Geometry check sheet. Reference: the model listing, model coordinates, mm. A direction names the side the tool comes from. Give positions to 0.01 mm unless a question says otherwise; leave off trailing zeros. Write each loop counter-clockwise with the first axis right and the second up, starting at its lowest first coordinate (ties: lowest second). Pieces come first, ordered by that corner, then holes. Notation, with made-up numbers: (37, 42) - (90, 42) arc R32 cw to (90, 71) - close; hole circle Ø2 at (-30, -25). An arc over 180 degrees is marked (long way). Use a Markdown table: item, result.
```python
from build123d import *
from build123d import SkipClean  # not in build123d's __all__

# Parameters (mm, degrees)
F0_W          = 30
F0_H          = 37
F0_W_2        = 3
F0_H_2        = 35
F1_DEPTH      = 32
F2_DEPTH      = 25
F3_W          = 3
F3_H          = 35
F4_DEPTH      = 30
F5_W          = 11.5
F5_H          = 11.5
F6_DEPTH      = 2
F5_R          = 2.5
F7_DEPTH      = 25
F8_T4_DEPTH   = 21.8227903205
F8_T9_DEPTH   = 21.8227903205
F8_T14_DEPTH  = 21.8227903205
F8_T19_DEPTH  = 21.8227903205
F9_R          = 7.5
F9_R_2        = 2.5
F10_DEPTH     = 3
F11_SIZE      = 2.99999
F12_W         = 11.5
F12_H         = 11.5
F13_DEPTH     = 2
F14_T4_DEPTH  = 21.8227903205
F14_T9_DEPTH  = 21.8227903205
F14_T14_DEPTH = 21.8227903205
F14_T19_DEPTH = 21.8227903205
F12_R         = 2.5
F15_DEPTH     = 25
F16_R         = 7.5
F16_R_2       = 2.5
F17_DEPTH     = 3
F19_SIZE2     = 2.99999
F19_SIZE      = 1.99999
F19_2_SIZE2   = 2.99999
F19_2_SIZE    = 1.99999
F21_DEPTH     = 5
F22_R         = 1


# Not quite as in the source:
# - a fillet or chamfer that OpenCascade refuses, or shapes differently, is made with other operations: its cross-section is extruded or revolved along the edge and cut away or added
# - a fillet or chamfer is up to 0.001 mm smaller than in the source, because OpenCascade refuses the exact size
# - after a boolean that leaves OpenCascade's solid faulty, fix() repairs it


with BuildPart() as f1:
    # F0 (on Front) → F1 (new body)
    with BuildSketch(Plane.XZ):
        with Locations((3.5, 0)):
            Rectangle(F0_W, F0_H)
        Polygon((-18.5, -18.5), (-11.5, -18.5), (-11.5, 18.5), (-13.5, 18.5), (-13.5, -16.5), (-16.5, -16.5), (-16.5, 18.5), (-18.5, 18.5), align=None)
        with Locations((-15, 1)):
            Rectangle(F0_W_2, F0_H_2)
    extrude(amount=F1_DEPTH)

    # F0 (on Front) → F2 (cut)
    with BuildSketch(Plane.XZ):
        with Locations((3.5, 0)):
            Rectangle(F0_W, F0_H)
        with Locations((-15, 1)):
            Rectangle(F0_W_2, F0_H_2)
    extrude(amount=F2_DEPTH, mode=Mode.SUBTRACT)

    # F3 (on face) → F4 (cut)
    with BuildSketch(Plane.YZ.offset(18.5)):
        with Locations((-28.5, 1)):
            Rectangle(F3_W, F3_H)
    extrude(amount=-F4_DEPTH, mode=Mode.SUBTRACT)

    # F5 (on face) → F6 (join)
    with BuildSketch(Plane(origin=(0, -25, 0), x_dir=(-1, 0, 0), z_dir=(0, 1, 0))):
        with Locations((-3.5, 1)):
            Rectangle(F5_W, F5_H)
        Polygon((-8.1188021535, 1), (-5.8094010768, 5), (-1.1905989232, 5), (1.1188021535, 1), (-1.1905989232, -3), (-5.8094010768, -3), align=None, mode=Mode.SUBTRACT)
    extrude(amount=F6_DEPTH)

    # F5 (on face) → F7 (cut)
    with BuildSketch(Plane(origin=(0, -25, 0), x_dir=(-1, 0, 0), z_dir=(0, 1, 0))):
        with Locations((-3.5, 1)):
            Circle(F5_R)
    extrude(amount=-F7_DEPTH, mode=Mode.SUBTRACT)

    # F8: chamfer of 1.5 x 2 on 4 edges, made by hand


with BuildPart() as f8_tool2:
    # F8_s3 → F8_t4 (new body)
    with BuildSketch(Plane.XY.offset(11.9113951602)):
        Polygon((9.25, -25), (7.75, -23), (9.25, -23), align=None)
    extrude(amount=-F8_T4_DEPTH)

    split(bisect_by=Plane.XZ.offset(25), keep=Keep.BOTTOM)


with BuildPart() as f1_1:
    add(f1.part, clean=False)

    # F8_t1: cut F8_tool2
    add(f8_tool2.part, mode=Mode.SUBTRACT)


with BuildPart() as f8_tool7:
    # F8_s8 → F8_t9 (new body)
    with BuildSketch(Plane.YZ.offset(-7.4113951602)):
        Polygon((-25, 6.75), (-23, 5.25), (-23, 6.75), align=None)
    extrude(amount=F8_T9_DEPTH)

    split(bisect_by=Plane.XZ.offset(25), keep=Keep.BOTTOM)


with BuildPart() as f1_2:
    add(f1_1.part, clean=False)

    # F8_t6: cut F8_tool7
    add(f8_tool7.part, mode=Mode.SUBTRACT)


with BuildPart() as f8_tool12:
    # F8_s13 → F8_t14 (new body)
    with BuildSketch(Plane.XY.offset(-9.9113951602)):
        Polygon((-2.25, -25), (-0.75, -23), (-2.25, -23), align=None)
    extrude(amount=F8_T14_DEPTH)

    split(bisect_by=Plane.XZ.offset(25), keep=Keep.BOTTOM)


with BuildPart() as f1_3:
    add(f1_2.part, clean=False)

    # F8_t11: cut F8_tool12
    add(f8_tool12.part, mode=Mode.SUBTRACT)


with BuildPart() as f8_tool17:
    # F8_s18 → F8_t19 (new body)
    with BuildSketch(Plane.YZ.offset(14.4113951602)):
        Polygon((-25, -4.75), (-23, -3.25), (-23, -4.75), align=None)
    extrude(amount=-F8_T19_DEPTH)

    split(bisect_by=Plane.XZ.offset(25), keep=Keep.BOTTOM)


with BuildPart() as f1_4:
    add(f1_3.part, clean=False)

    # F8_t16: cut F8_tool17
    add(f8_tool17.part, mode=Mode.SUBTRACT)

    # F9 (on face) → F10 (join)
    with BuildSketch(Plane.XZ.offset(32)):
        with Locations((3.5, 1)):
            Circle(F9_R)
        with Locations((3.5, 1)):
            Circle(F9_R_2, mode=Mode.SUBTRACT)
    with SkipClean():  # cleaning this boolean's faces spoils the solid; the shape is the same uncleaned
        extrude(amount=F10_DEPTH)

    # F11 (size 3 in the source; OpenCascade refuses exactly that, so slightly less here)
    f11_edges = [f1_4.edges().sort_by_distance(p)[0] for p in [
        (1, -35, 1),
    ]]
    chamfer(f11_edges, length=F11_SIZE)

    # F12 (on face) → F13 (join)
    with BuildSketch(Plane.YZ.offset(-11.5)):
        with Locations((-10, 1)):
            Rectangle(F12_W, F12_H)
        Polygon((-10, 5.6188021535), (-6, 3.3094010768), (-6, -1.3094010768), (-10, -3.6188021535), (-14, -1.3094010768), (-14, 3.3094010768), align=None, mode=Mode.SUBTRACT)
    extrude(amount=F13_DEPTH)

    add(f1_4.part.fix(), mode=Mode.REPLACE)

    # F14: chamfer of 1.5 x 2 on 4 edges, made by hand


with BuildPart() as f14_tool2:
    # F14_s3 → F14_t4 (new body)
    with BuildSketch(Plane.XY.offset(-9.9113951602)):
        Polygon((-11.5, -4.25), (-9.5, -5.75), (-9.5, -4.25), align=None)
    extrude(amount=F14_T4_DEPTH)

    split(bisect_by=Plane.YZ.offset(-11.5), keep=Keep.TOP)


with BuildPart() as f1_5:
    add(f1_4.part, clean=False)

    # F14_t1: cut F14_tool2
    add(f14_tool2.part, mode=Mode.SUBTRACT)


with BuildPart() as f14_tool7:
    # F14_s8 → F14_t9 (new body)
    with BuildSketch(Plane.XZ.offset(20.9113951602)):
        Polygon((-11.5, -4.75), (-9.5, -3.25), (-9.5, -4.75), align=None)
    extrude(amount=-F14_T9_DEPTH)

    split(bisect_by=Plane.YZ.offset(-11.5), keep=Keep.TOP)


with BuildPart() as f1_6:
    add(f1_5.part, clean=False)

    # F14_t6: cut F14_tool7
    add(f14_tool7.part, mode=Mode.SUBTRACT)


with BuildPart() as f14_tool12:
    # F14_s13 → F14_t14 (new body)
    with BuildSketch(Plane.XY.offset(11.9113951602)):
        Polygon((-11.5, -15.75), (-9.5, -14.25), (-9.5, -15.75), align=None)
    extrude(amount=-F14_T14_DEPTH)

    split(bisect_by=Plane.YZ.offset(-11.5), keep=Keep.TOP)


with BuildPart() as f1_7:
    add(f1_6.part, clean=False)

    # F14_t11: cut F14_tool12
    add(f14_tool12.part, mode=Mode.SUBTRACT)


with BuildPart() as f14_tool17:
    # F14_s18 → F14_t19 (new body)
    with BuildSketch(Plane.XZ.offset(-0.9113951602)):
        Polygon((-11.5, 6.75), (-9.5, 5.25), (-9.5, 6.75), align=None)
    extrude(amount=F14_T19_DEPTH)

    split(bisect_by=Plane.YZ.offset(-11.5), keep=Keep.TOP)


with BuildPart() as f1_8:
    add(f1_7.part, clean=False)

    # F14_t16: cut F14_tool17
    add(f14_tool17.part, mode=Mode.SUBTRACT)

    # F12 (on face) → F15 (cut)
    with BuildSketch(Plane.YZ.offset(-11.5)):
        with Locations((-10, 1)):
            Circle(F12_R)
    extrude(amount=-F15_DEPTH, mode=Mode.SUBTRACT)

    # F16 (on face) → F17 (join)
    with BuildSketch(Plane(origin=(-18.5, 0, 0), x_dir=(0, -1, 0), z_dir=(-1, 0, 0))):
        with Locations((10, 1)):
            Circle(F16_R)
        with Locations((10, 1)):
            Circle(F16_R_2, mode=Mode.SUBTRACT)
    extrude(amount=F17_DEPTH)

    # F18: chamfer of 3 on 1 edges, made by hand

    # F18_s1 → F18_t2 (revolve, cut)
    with BuildSketch(Plane.XY.offset(1)):
        Polygon((-18.5, -12.5), (-21.5, -15.5), (-21.5, -12.5), align=None)
    revolve(axis=Axis((-21.5, -10, 1), (-1, 0, 0)), mode=Mode.SUBTRACT)

    # F19 (size 2 and 3 in the source; OpenCascade refuses exactly that, so slightly less here)
    f19_edges = [f1_8.edges().sort_by_distance(p)[0] for p in [
        (-21.5, -2.5, 1),
    ]]
    f19_side = f1_8.faces().sort_by_distance((-21.5, -2.712132, 1))[0]
    chamfer(f19_edges, length=F19_SIZE, length2=F19_SIZE2, reference=f19_side)

    # F19#2 (size 2 and 3 in the source; OpenCascade refuses exactly that, so slightly less here)
    f19_2_edges = [f1_8.edges().sort_by_distance(p)[0] for p in [
        (-4, -35, 1),
    ]]
    f19_2_side = f1_8.faces().sort_by_distance((-2.212122, -35, 1))[0]
    chamfer(f19_2_edges, length=F19_2_SIZE, length2=F19_2_SIZE2, reference=f19_2_side)

    # F20 (on face) → F21 (join)
    with BuildSketch(Plane(origin=(0, 0, 0), x_dir=(-1, 0, 0), z_dir=(0, 1, 0))):
        Polygon((11.5, -4.75), (11.5, -18.5), (18.5, -18.5), (18.5, 18.5), (16.5, 18.5), (16.5, -16.5), (13.5, -16.5), (13.5, 18.5), (11.5, 18.5), (11.5, 6.75), align=None)
    extrude(amount=F21_DEPTH)

    # F22
    f22_edges = [f1_8.edges().sort_by_distance(p)[0] for p in [
        (-11.5, 5, 0),
        (-18.5, 5, 0),
        (-11.5, -10, -18.5),
        (3.5, -25, -18.5),
        (0, -32, -18.5),
        (18.5, -32, 0),
        (18.5, -25, 0),
        (-15, 5, -18.5),
        (-18.5, -13.5, -18.5),
        (18.5, -28.5, -18.5),
        (-18.5, -32, 0),
    ]]
    fillet(f22_edges, radius=F22_R)


solid = f1_8.part
```
1) Section check D-D on y = -19.5. Record the boundary of the cut face in (x, z).
Working result:
| item | result |
|---|---|
| outline | (-18.5, -17.5) arc R1 ccw to (-17.5, -18.5) - (-12.5, -18.5) arc R1 ccw to (-11.5, -17.5) - (-11.5, 18.5) - (-13.5, 18.5) - (-13.5, -16.5) - (-16.5, -16.5) - (-16.5, 18.5) - (-18.5, 18.5) - close |
2) Section check C-C on z = -14. Record the boundary of the cut face in (x, y), then the cut area to 3 significant figures.
Working result:
| item | result |
|---|---|
| outline | (-18.5, -31) arc R1 ccw to (-17.5, -32) - (17.5, -32) arc R1 ccw to (18.5, -31) - (18.5, -30) - (-11.5, -30) - (-11.5, -27) - (18.5, -27) - (18.5, -26) arc R1 ccw to (17.5, -25) - (-11.5, -25) - (-11.5, 4) arc R1 ccw to (-12.5, 5) - (-13.5, 5) - (-13.5, -25) - (-16.5, -25) - (-16.5, 5) - (-17.5, 5) arc R1 ccw to (-18.5, 4) - close |
| area | 288 mm² |
3) Set-up check for faces 1 (the flat face through (3, -24, -3)), 2 (the flat face through (-10.5, -9.9, 6)), 3 (the flat face through (7, -30, 1)), 4 (the flat face through (-10.514, -7.972, -2.448)): record each of +Z, -Z, +X, -X, +Y, -Y from which the full face is reachable in a straight line by a thin tool's end or side.
Working result:
| item | result |
|---|---|
| face 1 | +Y |
| face 2 | +Z, +X, +Y |
| face 3 | +Z, +X |
| face 4 | +X |
4) Mould release check, pull along X, two halves, no side actions. Record for faces 5 (the flat face through (-10.514, -12.028, 4.448)), 6 (the flat face through (-10.5, -5, 0.9)), 7 (the flat face through (0.02, -24.01, -0.97)): pulls with the +X half, pulls with the -X half, needs draft (parallel to the pull), parting line crosses it, or undercut.
Working result:
| item | result |
|---|---|
| face 5 | needs draft |
| face 6 | pulls with the +X half |
| face 7 | undercut |
5) Depth check by flat-ended pin: P1, Ø8, axis at y = -27, z = 12.5, coming from the -X side; P2, Ø1.8, axis at x = 4.5, z = -2, coming from the +Y side; P3, Ø10, axis at x = -7, y = -9.5, coming from the -Z side; P4, Ø15, axis at y = -7.5, z = 0, coming from the -X side. Enter the tip coordinate at first touch or a pass-through.
Working result:
| item | result |
|---|---|
| P1 | stops at x = -18.5 |
| P2 | stops at y = -25 |
| P3 | stops at z = -18.37 |
| P4 | stops at x = -21.5 |
6) Section check B-B on y = -29. Record the boundary of the cut face in (x, z), then the cut area to 3 significant figures.
Working result:
| item | result |
|---|---|
| outline | (-18.5, -17.5) arc R1 ccw to (-17.5, -18.5) - (17.5, -18.5) arc R1 ccw to (18.5, -17.5) - (18.5, -16.5) - (-11.5, -16.5) - (-11.5, 18.5) - (-18.5, 18.5) - close |
| area | 319 mm² |
7) Material ranges on L1, parallel to X at y = -18.5, z = 14; L2, parallel to Y at x = 10, z = -11.5; L3, parallel to Z at x = 3.5, y = -26.1, recorded low to high. Write a range as from..to.
Working result:
| item | result |
|---|---|
| L1 | x = -18.5..-16.5, -13.5..-11.5 |
| L2 | y = -32..-30, -27..-25 |
| L3 | z = -18.5..-1.5, 3.5..18.5 |
8) Section check A-A on x = 3.5. Count the separate pieces of the cut face and the enclosed holes in it, then the cut area to 3 significant figures.
Working result:
| item | result |
|---|---|
| separate pieces | 3 |
| enclosed holes | 0 |
| area | 153 mm² |
